Can you work these out from the model? Positions are in its coordinate system, mm. Face numbers are marked on the shaded views. Round coordinates to 2 decimals unless told otherwise and drop trailing zeros. Loops run counter-clockwise (first coordinate to the right, second up) from the corner with the lowest first, then second, coordinate; pieces in that order, holes last. Notation, with made-up numbers: (74.5, 61) - (92.5, 61) arc R6 ccw to (92.5, 66) - close; hole circle Ø1 at (81.25, 17). An arc over 180 degrees is marked (long way). Answer as CSV lines item,"result".
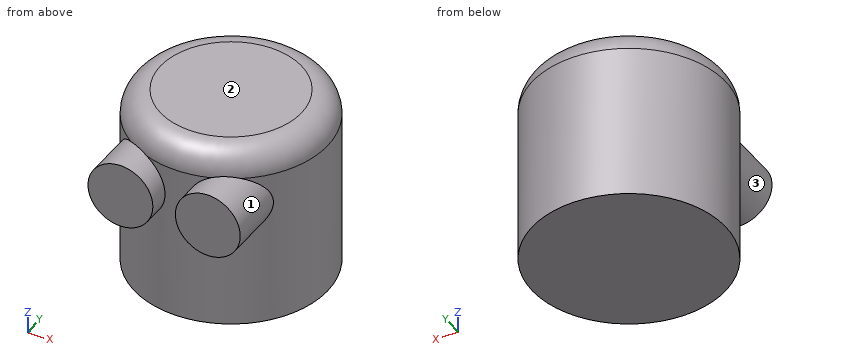
```python
from build123d import *

# Parameters (mm, degrees)
F0_R     = 37.091659
F1_DEPTH = 70
F2_R     = 10
F3_R     = 12.5
F4_DEPTH = 45


with BuildPart() as f1:
    # F0 (on Top) → F1 (new body)
    with BuildSketch(Plane.XY):
        Circle(F0_R)
    extrude(amount=F1_DEPTH)

    # F2
    f2_edges = [f1.edges().sort_by_distance(p)[0] for p in [
        (-37.091659, 0, 70),
    ]]
    fillet(f2_edges, radius=F2_R)

    # F3 (on Front) → F4 (join)
    with BuildSketch(Plane.XZ):
        with Locations((-16.831745, 48.336694)):
            Circle(F3_R)
        with Locations((16.831745, 48.336694)):
            Circle(F3_R)
    extrude(amount=F4_DEPTH)


solid = f1.part
```
Q1. If I drill on line 1 along X through (y, z) = (-1, 23); line 2 along Y through (x, z) = (-29, 54.5); line 3 along Y through (x, z) = (-28.5, 44.5), over which ranges is the centre line in solid material (lowest first)? Write a range as [from, to].
Checks:
line 1,"[-37.08, 37.08]"
line 2,"[-23.13, 23.13]"
line 3,"[-45, 23.74]"
Q2. Imagine slicing it at A-A (x = 0). Write out the boundary of the cut face in (y, z), then the cut area to 3 significant figures.
Checks:
outline,"(-37.09, 0) - (37.09, 0) - (37.09, 60) arc R10 ccw to (27.09, 70) - (-27.09, 70) arc R10 ccw to (-37.09, 60) - close"
area,"5,150 mm²"
Q3. We'd pull the mould along X, two halves only. Please class the marked faces 1, 2 and 3: pulls with the +X half, pulls with the -X half, needs draft (parallel to the pull), parting line crosses it, or undercut.
Checks:
face 1,"undercut"
face 2,"needs draft"
face 3,"undercut"
Q4. I'm going to push flat-ended pins straight in: pin 1 Ø1 at (x, z) = (22.5, 40.5) entering from +Y; pin 2 Ø1 at (y, z) = (-15.5, 34.5) entering from +X; pin 3 Ø5 at (y, z) = (-29, 55.5) entering from +X. Where does each tip first touch, or does it pass through?
Checks:
pin 1,"y = 29.86"
pin 2,"x = 33.92"
pin 3,"x = 28.43"
